```python
from build123d import *

# Parameters (mm, degrees)
TUBE_SQUARE_TS3X3X0_3125_1_DEPTH = 1450
SKETCH7_R                        = 5
CUT_EXTRUDE1_DEPTH               = 742.636703515


with BuildPart() as part:
    # Sketch1 → Tube square TS3X3X0.3125(1) (new body)
    with BuildSketch(Plane(origin=(0, 0, -725), x_dir=(0, -1, 0), z_dir=(0, 0, 1))):
        with BuildLine():
            Line((-90, -60), (90, -60))
            ThreePointArc((90, -60), (97.071067812, -57.071067812), (100, -50))
            Line((100, -50), (100, 50))
            ThreePointArc((100, 50), (97.071067812, 57.071067812), (90, 60))
            Line((90, 60), (-90, 60))
            ThreePointArc((-90, 60), (-97.071067812, 57.071067812), (-100, 50))
            Line((-100, 50), (-100, -50))
            ThreePointArc((-100, -50), (-97.071067812, -57.071067812), (-90, -60))
        make_face()
        with BuildLine():
            Line((-90, -52), (90, -52))
            ThreePointArc((90, -52), (91.414213562, -51.414213562), (92, -50))
            Line((92, -50), (92, 50))
            ThreePointArc((92, 50), (91.414213562, 51.414213562), (90, 52))
            Line((90, 52), (-90, 52))
            ThreePointArc((-90, 52), (-91.414213562, 51.414213562), (-92, 50))
            Line((-92, 50), (-92, -50))
            ThreePointArc((-92, -50), (-91.414213562, -51.414213562), (-90, -52))
        make_face(mode=Mode.SUBTRACT)
    extrude(amount=TUBE_SQUARE_TS3X3X0_3125_1_DEPTH)

    # Sketch7 → Cut-Extrude1 (cut, through all)
    with BuildSketch(Plane(origin=(60, 0, 0), x_dir=(0, 0, -1), z_dir=(1, 0, 0))):
        with Locations(Location((647, 0, 0), (0, 0, 90))):
            Circle(SKETCH7_R)
        with Locations(Location((447, 0, 0), (0, 0, 90))):
            Circle(SKETCH7_R)
        with Locations(Location((247, 0, 0), (0, 0, 90))):
            Circle(SKETCH7_R)
        with Locations(Location((47, 0, 0), (0, 0, 90))):
            Circle(SKETCH7_R)
        with Locations(Location((-153, 0, 0), (0, 0, 90))):
            Circle(SKETCH7_R)
        with Locations(Location((-353, 0, 0), (0, 0, 90))):
            Circle(SKETCH7_R)
        with Locations(Location((-553, 0, 0), (0, 0, 90))):
            Circle(SKETCH7_R)
    extrude(amount=-CUT_EXTRUDE1_DEPTH, mode=Mode.SUBTRACT)


solid = part.part
```
CAD build for the part. Positions are in the model's coordinates, mm. A direction names the side the tool comes from. Coordinates: 2 decimals unless noted, no trailing zeros. Write each loop counter-clockwise with the first axis right and the second up, starting at its lowest first coordinate (ties: lowest second). Pieces come first, ordered by that corner, then holes.
(1) Cut at B-B, the plane x = 2. List the corners of the cut face in (y, z).
(2) Cut at A-A, the plane y = -42. List the corners of the cut face in (x, z), and give its area (3 significant figures).
(3) 3-axis set-ups, long thin cutter, end or side, ignore diameter. For faces 1 (the face through (-52, 1, -10)), 2 (the face through (-53, 0, -725)): which of +Z, -Z, +X, -X, +Y, -Y reach the whole face in a straight line?
(4) Drill centre lines: probe 1 along Y at (x, z) = (37, 528.5); probe 2 along X at (y, z) = (-80.5, 536.5); probe 3 along Y at (x, z) = (-53.75, -647). Where is each one in solid material? Low to high.
(5) Cut at C-C, the plane z = 295.5. List the corners of the cut face in (x, y).
(6) Flat gauge pin, fed straight in: pin 1 (8 mm diameter, centred on y = 0, z = -647, fed in from +X). Where does the tip first touch, or does it go through?
(7) Two-plate mould, pull along Y, no slides. Class faces 3 (the face through (52, -1, -10)), 4 (the face through (-1, -100, -10)), 5 (the face through (1, 100, -10)): +Y half, -Y half, draft (parallel to the pull), parting line (faces both ways), or undercut.
Geometry says:
1. outline: (-100, -725) - (-92, -725) - (-92, 725) - (-100, 725) - close; (92, -725) - (100, -725) - (100, 725) - (92, 725) - close
2. outline: (-60, -725) - (-52, -725) - (-52, 725) - (-60, 725) - close; (52, -725) - (60, -725) - (60, 725) - (52, 725) - close
2. area: 23,200 mm2
3. face 1: +Z, -Z
3. face 2: -Z, +X, -X, +Y, -Y
4. probe 1: y = -100 to -92, 92 to 100
4. probe 2: x = -60 to -52, 52 to 60
4. probe 3: y = -99.27 to -5, 5 to 99.27
5. outline: (-60, -90) arc R10 ccw to (-50, -100) - (50, -100) arc R10 ccw to (60, -90) - (60, 90) arc R10 ccw to (50, 100) - (-50, 100) arc R10 ccw to (-60, 90) - close; hole (-52, -90) arc R2 ccw to (-50, -92) - (50, -92) arc R2 ccw to (52, -90) - (52, 90) arc R2 ccw to (50, 92) - (-50, 92) arc R2 ccw to (-52, 90) - close
6. pin 1: passes through
7. face 3: undercut
7. face 4: -Y half
7. face 5: +Y half
